For this review, take the finished solid that the model builds, in its own axes (mm). Face numbers are marked on the shaded views. A direction names the side the tool comes from. Round coordinates to 2 decimals unless told otherwise and drop trailing zeros. Order: outer loops, then holes, each group sorted by start corner. A loop starts at its lowest first (then second) coordinate and runs counter-clockwise, first axis right, second up.
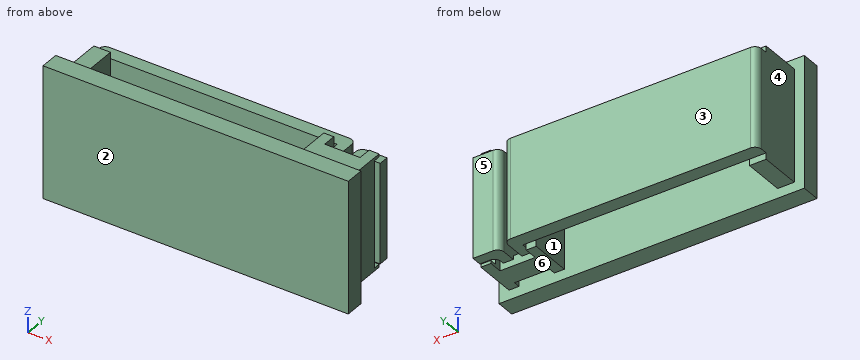
```python
from build123d import *

# Parameters (mm, degrees)
BASE_OUTLINE_W              = 45.8
BASE_OUTLINE_H              = 19.8
CLAMP_BASE_DEPTH            = 2.8
HINGE_AND_LATCH_OUTLINE_W   = 2.5
HINGE_AND_LATCH_OUTLINE_H   = 6.2
HINGE_AND_LATCH_OUTLINE_W_2 = 8.3
CLIP_HINGE_AND_LATCH_DEPTH  = 8.45
LATCH_SIDES_CUT_REACH       = 32.694
SIDE_CUTS_OUTLINE_W         = 5.3
SIDE_CUTS_OUTLINE_H         = 2
SIDE_CUTS_OUTLINE_H_2       = 1
LATCH_THROUGH_CUT_REACH     = 27.912
THROUGH_CUT_OUTLINE_W       = 5.3
THROUGH_CUT_OUTLINE_H       = 13.9
LATCH_FRONT_CUT_REACH       = 48.276
FRONT_CUT_OUTLINE_W         = 16
FRONT_CUT_OUTLINE_H         = 1
CLAMP_DEPTH                 = 7.5
CLAMP_FILLETS_R             = 1


with BuildPart() as part:
    # Base Outline → Clamp Base (new body)
    with BuildSketch(Plane(origin=(0, 0, 0), x_dir=(1, 0, 0), z_dir=(0, 1, 0))):
        Rectangle(BASE_OUTLINE_W, BASE_OUTLINE_H)
    extrude(amount=CLAMP_BASE_DEPTH)

    # Hinge and Latch Outline → Clip Hinge and Latch (add, symmetric)
    with BuildSketch(Plane.XY):
        with Locations((-20.15, 5.9)):
            Rectangle(HINGE_AND_LATCH_OUTLINE_W, HINGE_AND_LATCH_OUTLINE_H)
        with Locations((17.25, 5.9)):
            Rectangle(HINGE_AND_LATCH_OUTLINE_W_2, HINGE_AND_LATCH_OUTLINE_H)
    extrude(amount=CLIP_HINGE_AND_LATCH_DEPTH, both=True)

    # Side Cuts Outline → Latch Sides Cut (cut, up to next)
    with BuildSketch(Plane.XY.offset(8.45), mode=Mode.PRIVATE) as latch_sides_cut_sk1:
        with Locations((17.25, 8)):
            Rectangle(SIDE_CUTS_OUTLINE_W, SIDE_CUTS_OUTLINE_H)
    latch_sides_cut_tool1 = extrude(latch_sides_cut_sk1.sketch, amount=-LATCH_SIDES_CUT_REACH, mode=Mode.PRIVATE) & part.part
    # Side Cuts Outline → Latch Sides Cut (cut, up to next)
    with BuildSketch(Plane.XY.offset(8.45), mode=Mode.PRIVATE) as latch_sides_cut_sk2:
        with Locations((17.25, 3.3)):
            Rectangle(SIDE_CUTS_OUTLINE_W, SIDE_CUTS_OUTLINE_H_2)
    latch_sides_cut_tool2 = extrude(latch_sides_cut_sk2.sketch, amount=-LATCH_SIDES_CUT_REACH, mode=Mode.PRIVATE) & part.part
    add(latch_sides_cut_tool1.solids().sort_by_distance((17.25, 8, 8.45))[0], mode=Mode.SUBTRACT)
    add(latch_sides_cut_tool2.solids().sort_by_distance((17.25, 3.3, 8.45))[0], mode=Mode.SUBTRACT)

    # Through Cut Outline → Latch Through Cut (cut, up to next)
    with BuildSketch(Plane(origin=(0, 7, 0), x_dir=(1, 0, 0), z_dir=(0, 1, 0)), mode=Mode.PRIVATE) as latch_through_cut_sk1:
        with Locations((17.25, 0)):
            Rectangle(THROUGH_CUT_OUTLINE_W, THROUGH_CUT_OUTLINE_H)
    latch_through_cut_tool1 = extrude(latch_through_cut_sk1.sketch, amount=-LATCH_THROUGH_CUT_REACH, mode=Mode.PRIVATE) & part.part
    add(latch_through_cut_tool1.solids().sort_by_distance((17.25, 7, 0))[0], mode=Mode.SUBTRACT)

    # Front Cut Outline → Latch Front Cut (cut, up to next)
    with BuildSketch(Plane(origin=(21.4, 0, 0), x_dir=(0, 0, -1), z_dir=(1, 0, 0)), mode=Mode.PRIVATE) as latch_front_cut_sk1:
        with Locations((0, 8.5)):
            Rectangle(FRONT_CUT_OUTLINE_W, FRONT_CUT_OUTLINE_H)
    latch_front_cut_tool1 = extrude(latch_front_cut_sk1.sketch, amount=-LATCH_FRONT_CUT_REACH, mode=Mode.PRIVATE) & part.part
    add(latch_front_cut_tool1.solids().sort_by_distance((21.4, 8.5, 0))[0], mode=Mode.SUBTRACT)

    # Clamp Outline → Clamp (add, symmetric)
    with BuildSketch(Plane.XY):
        Polygon((-21.4, 9), (15.1, 9), (15.1, 3.3), (19.4, 3.3), (19.4, 8.5), (21.9, 8.5), (21.9, 10), (17.9, 10), (17.9, 4.8), (16.6, 4.8), (16.6, 11), (-21.4, 11), align=None)
    extrude(amount=CLAMP_DEPTH, both=True)

    # Clamp Fillets
    clamp_fillets_edges = [part.edges().sort_by_distance(p)[0] for p in [
        (19.4, 8.5, 0),
        (17.9, 10, 0),
        (16.6, 11, 0),
        (-21.4, 11, 0),
        (19.4, 3.3, 0),
        (15.1, 3.3, 0),
    ]]
    fillet(clamp_fillets_edges, radius=CLAMP_FILLETS_R)


solid = part.part
```
Q1. Tool access review of the marked faces 4, 5 and 6: name each direction out of +Z, -Z, +X, -X, +Y, -Y from which nothing blocks a thin tool from reaching the whole face with its end or side.
Q2. Clearance check with flat-ended pins moving along their axes: pin 1 (0.5 mm diameter, centred on x = 14, z = 8, fed in from +Y); pin 2 (3 mm diameter, centred on y = 4.5, z = 3, fed in from +X); pin 3 (2 mm diameter, centred on y = 9.5, z = 7.5, fed in from -X); pin 4 (3 mm diameter, centred on x = -1.5, y = 4.5, fed in from -Z). State where each tip first meets the part, or that it passes through.
Q3. Mouldability with a two-part tool opening along Y and no side actions: class the marked faces 1, 2 and 3 as +Y half, -Y half, draft (parallel to the pull), parting line (faces both ways), or undercut.
Q4. Take a section at A-A, the plane y = 5.25. State the section outline as (x, z) points, plus the area to 3 significant figures.
Q5. Wall thickness on line 1 (X direction, y = 4.75, z = -7); line 2 (Y direction, x = 7, z = 3.5); line 3 (X direction, y = 5.25, z = -4.75): over which ranges is each line inside the solid? List them lowest first.
Q6. Take a section at B-B, the plane x = 4. State the section outline as (y, z) points.
Working result:
1. face 4: +Z, -Z, -X, +Y
1. face 5: +Z, -Z, +X, +Y
1. face 6: -Z, +X, -X, +Y
2. pin 1: stops at y = 9
2. pin 2: stops at x = 21.4
2. pin 3: stops at x = -21.4
2. pin 4: passes through
3. face 1: undercut
3. face 2: -Y half
3. face 3: +Y half
4. outline: (-21.4, -8.45) - (-18.9, -8.45) - (-18.9, 8.45) - (-21.4, 8.45) - close; (13.1, -8.45) - (21.4, -8.45) - (21.4, 8.45) - (13.1, 8.45) - close; hole (14.6, -6.95) - (15.1, -6.95) - (15.1, 6.95) - (14.6, 6.95) - close; hole (16.6, -6.95) - (17.9, -6.95) - (17.9, 6.95) - (16.6, 6.95) - close; hole (19.4, -6.95) - (19.9, -6.95) - (19.9, 6.95) - (19.4, 6.95) - close
4. area: 151 mm2
5. line 1: x = -21.4 to -18.9, 13.1 to 21.4
5. line 2: y = 0 to 2.8, 9 to 11
5. line 3: x = -21.4 to -18.9, 13.1 to 14.6, 15.1 to 16.6, 17.9 to 19.4, 19.9 to 21.4
6. outline: (0, -9.9) - (2.8, -9.9) - (2.8, 9.9) - (0, 9.9) - close; (9, -7.5) - (11, -7.5) - (11, 7.5) - (9, 7.5) - close
